```python
from build123d import *

# Parameters (mm, degrees)
HOLE_WIZARD_1_4_1_D      = 7.14248
PATTERN_CIRCULAR_1_COUNT = 4
SKETCH_6_W               = 10
SKETCH_6_H               = 20
EXTRUDE_1_DEPTH          = 85
SKETCH_7_W               = 50
SKETCH_7_H               = 20
EXTRUDE_2_DEPTH          = 5


with BuildPart() as part:
    # Sketch 1 → Revolve 1 (revolve)
    with BuildSketch(Plane(origin=(0, 0, 0), x_dir=(1, 0, 0), z_dir=(0, 1, 0)), mode=Mode.PRIVATE) as revolve_1_sk:
        Polygon((111.732704886, 39.491362749), (116.090992439, 39.491362749), (116.090992439, 37.435413944), (112.5, 35.478273614), (112.5, -34.508637251), (145.5, -34.508637251), (145.5, -40.508637251), (112.5, -40.508637251), (112.5, -60.508637251), (109.5, -60.508637251), (109.5, -54.831811372), (76.899138585, -54.831811372), (76.899138585, -48.831811372), (109.5, -48.831811372), (109.5, 35.478273614), (101.192673018, 42.998947767), (107.858230993, 42.998947767), align=None)
    revolve(revolve_1_sk.sketch.rotate(Axis((0, 0, -66.031649095), (0, 0, 1)), 180), axis=Axis((0, 0, -66.031649095), (0, 0, 1)))

    # Hole Wizard 1_4 _1 (through all)
    with Locations(Plane(origin=(-125.185676655, 51.853605085, 34.508637251), x_dir=(-1, 0, 0), z_dir=(0, 0, -1))):
        with Locations((0, 0), (0, -103.70721017)):
            hole_wizard_1_4_1 = Hole(HOLE_WIZARD_1_4_1_D / 2)

    # Pattern Circular 1: Hole Wizard 1_4 _1 ×4 about axis
    pattern_circular_1_axis = Axis((0, 0, 0), (0, 0, 1))
    for i in range(1, PATTERN_CIRCULAR_1_COUNT):
        add(hole_wizard_1_4_1.rotate(pattern_circular_1_axis, i * 360 / PATTERN_CIRCULAR_1_COUNT), mode=Mode.SUBTRACT)

    # Sketch 6 → Extrude 1 (add)
    with BuildSketch(Plane(origin=(0, 0, 48.831811372), x_dir=(-1, 0, 0), z_dir=(0, 0, -1))):
        Polygon((-31.397465716, -74.248707787), (-36.397465716, -82.908961825), (-53.717973792, -72.908961825), (-48.717973792, -64.248707787), align=None)
        with Locations((85, -0.066649031)):
            Rectangle(SKETCH_6_W, SKETCH_6_H)
        Polygon((-48.602534284, 64.315356818), (-53.602534284, 72.975610856), (-36.282026208, 82.975610856), (-31.282026208, 74.315356818), align=None)
    extrude(amount=EXTRUDE_1_DEPTH)

    # Sketch 7 → Extrude 2 (add)
    with BuildSketch(Plane(origin=(0, 0, -36.168188628), x_dir=(-1, 0, 0), z_dir=(0, 0, -1))):
        Polygon((-11.397465716, -39.607691636), (-36.397465716, -82.908961825), (-53.717973792, -72.908961825), (-28.717973792, -29.607691636), align=None)
        with Locations((65, -0.066649031)):
            Rectangle(SKETCH_7_W, SKETCH_7_H)
        Polygon((-28.602534284, 29.674340667), (-53.602534284, 72.975610856), (-36.282026208, 82.975610856), (-11.282026208, 39.674340667), align=None)
    extrude(amount=EXTRUDE_2_DEPTH)


solid = part.part
```
The model under review builds one solid part; all positions refer to its coordinate system, in mm. A direction names the side the tool comes from. Give positions to 0.01 mm unless a question says otherwise; leave off trailing zeros. Loops run counter-clockwise (first coordinate to the right, second up) from the corner with the lowest first, then second, coordinate; pieces in that order, holes last. Notation, with made-up numbers: (-21.5, -20.75) - (-1.5, -20.75) arc R33 ccw to (-1.5, 17.25) - close; hole circle Ø9 at (-18.75, -11.75). An arc over 180 degrees is marked (long way). Answer as a JSON object with one key per item and string values.
Q1. Insertion check: pin 1 (10 mm diameter, centred on x = 94, z = -22, fed in from -Y); pin 2 (9.5 mm diameter, centred on x = 125.19, y = -51.85, fed in from -Z); pin 3 (6 mm diameter, centred on y = 0, z = 13.5, fed in from +X). Each pin has a flat end and moves straight along its axis. Give the tip position at first contact, or say it passes through.
Worked out:
{"pin 1": "stops at y = -68.81", "pin 2": "stops at z = 34.51", "pin 3": "stops at x = 112.5"}
Q2. Add section A-A on z = -5. State the section outline as (x, y) points, plus the area to 3 significant figures.
Worked out:
{"outline": "circle Ø225 at (0, 0); (-90, -10.07) - (-80, -10.07) - (-80, 9.93) - (-90, 9.93) - close; (31.28, 74.32) - (48.6, 64.32) - (53.6, 72.98) - (36.28, 82.98) - close; (31.4, -74.25) - (36.4, -82.91) - (53.72, -72.91) - (48.72, -64.25) - close; hole circle Ø219 at (0, 0)", "area": "2,690 mm^2"}
Q3. To check wall thickness, follow line 1 along X through (y, z) = (-69, 11) (1 decimal); line 2 along Y through (x, z) = (45.5, 34); line 3 along Y through (x, z) = (0, -7). State the ranges of each line that lie inside material, in increasing order.
Worked out:
{"line 1": "x = -88.9 to -85, 40.5 to 51.5, 85 to 88.9", "line 2": "y = -102.89 to -99.6, -77.65 to -66.11, 66.11 to 77.65, 99.6 to 102.89", "line 3": "y = -112.5 to -109.5, 109.5 to 112.5"}
Q4. Mouldability with a two-part tool opening along Y and no side actions: class faces 1 (the cylindrical face through (127.818, -54.267, 37.551)), 2 (the cylindrical face through (-107.305, -33.792, 0.005)), 3 (the flat face through (-75, 86, 40.509)) as +Y half, -Y half, draft (parallel to the pull), parting line (faces both ways), or undercut.
Worked out:
{"face 1": "undercut", "face 2": "parting line", "face 3": "draft"}
Q5. Add section C-C on y = -60.5. Count the separate pieces of the cut face and the enclosed holes in it, plus the area to 3 significant figures.
Worked out:
{"separate pieces": "3", "enclosed holes": "0", "area": "1,910 mm^2"}
Q6. For faces 4 (the cylindrical face through (23.737, 106.896, 57.63)), 5 (the flat face through (45.064, 77.906, 4.462)), 6 (the cylindrical face through (23.737, 106.896, 6.087)), 7 (the cylindrical face through (-53.221, 121.887, 37.551)), list the 3-axis set-ups (+Z, -Z, +X, -X, +Y, -Y) from which the entire face can be reached by the end or side of a thin tool; tool diameter is ignored.
Worked out:
{"face 4": "+Z", "face 5": "-Z", "face 6": "none", "face 7": "+Z, -Z"}
